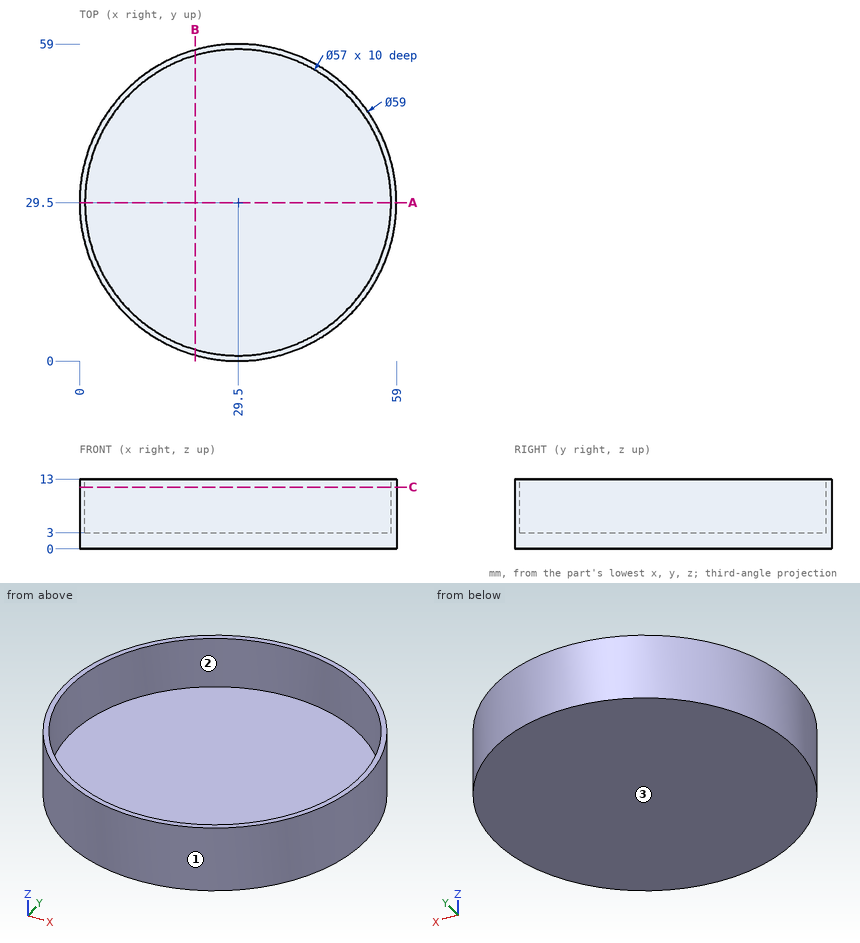
The figure shows three views and two pictorial views of one solid part (mm, origin at its lowest corner). Answer the questions. Coordinates: 2 decimals unless noted, no trailing zeros. Write each loop counter-clockwise with the first axis right and the second up, starting at its lowest first coordinate (ties: lowest second). Pieces come first, ordered by that corner, then holes.
1. Flat-ended cylindrical pins translate along their axes: pin 1 (2 mm diameter, centred on y = 35.5, z = 3.5, fed in from -X); pin 2 (3 mm diameter, centred on x = 36, z = 11.5, fed in from +Y); pin 3 (1.5 mm diameter, centred on y = 53, z = 11.5, fed in from -X). Find the tip coordinate at first contact, or state that the pin passes through.
Results list:
pin 1: stops at x = 0.43
pin 2: stops at y = 58.57
pin 3: stops at x = 10.72
2. Consider line 1 along Y through (x, z) = (29.5, 7.5); line 2 along Z through (x, y) = (13, 46); line 3 along Y through (x, z) = (16, 10.75). Determine where each line is inside the solid, lowest interval first.
Results list:
line 1: y = 0 to 1, 58 to 59
line 2: z = 0 to 3
line 3: y = 3.27 to 4.4, 54.6 to 55.73
3. The part is cut by section C-C, the plane z = 11.5. Write down the section's boundary in (x, y), and give its area (3 significant figures).
Results list:
outline: circle Ø59 at (29.5, 29.5); hole circle Ø57 at (29.5, 29.5)
area: 182 mm2
4. The part is cut by section B-B, the plane x = 21.5. Write down the section's boundary in (y, z), and give its area (3 significant figures).
Results list:
outline: (1.11, 0) - (57.89, 0) - (57.89, 13) - (56.85, 13) - (56.85, 3) - (2.15, 3) - (2.15, 13) - (1.11, 13) - close
area: 191 mm2
5. For a pull along X with two mould halves and no side action, classify the marked faces 1, 2 and 3 as +X half, -X half, draft (parallel to the pull), parting line (faces both ways), or undercut.
Results list:
face 1: parting line
face 2: undercut
face 3: draft
6. The part is cut by section A-A, the plane y = 29.5. Write down the section's boundary in (x, z).
Results list:
outline: (0, 0) - (59, 0) - (59, 13) - (58, 13) - (58, 3) - (1, 3) - (1, 13) - (0, 13) - close
